Check sheet for the modelled part. Datum: model origin and axes. Units: mm. Face numbers are marked on the shaded views. Give positions to 0.01 mm unless a question says otherwise; leave off trailing zeros. Write each loop counter-clockwise with the first axis right and the second up, starting at its lowest first coordinate (ties: lowest second). Pieces come first, ordered by that corner, then holes. Notation, with made-up numbers: (-35.5, 20.25) -> (15.5, 20.25) arc R28 ccw to (15.5, 49.25) -> close; hole circle Ø1 at (47, 68). An arc over 180 degrees is marked (long way). Return JSON: item names as keys, results as strings.
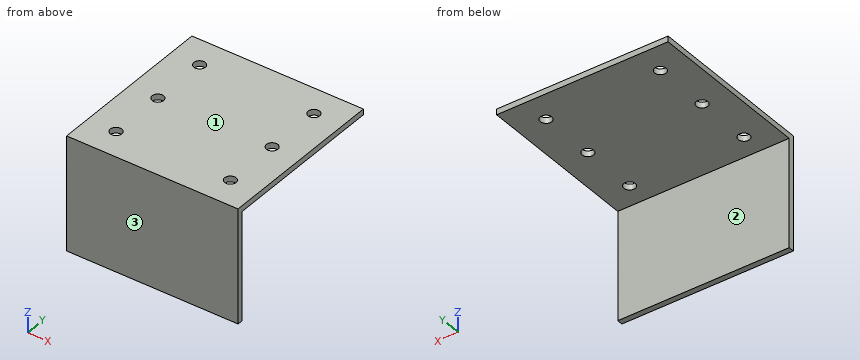
from build123d import *

# Parameters (mm, degrees)
EXTRUDE_1_DEPTH     = 60
SKETCH_2_R          = 2
CUT_EXTRUDE_1_DEPTH = 41


with BuildPart() as part:
    # Эскиз1 → Вытянуть-Тонкостенный1 (new body)
    with BuildSketch(Plane(origin=(0, 0, 0), x_dir=(0, 0, -1), z_dir=(1, 0, 0))):
        Polygon((40, 0), (0, 0), (0, 60), (2, 60), (2, 2), (40, 2), align=None)
    extrude(amount=EXTRUDE_1_DEPTH)

    # Эскиз2 → Вырез-Вытянуть1 (cut, through all)
    with BuildSketch(Plane.XY):
        with Locations((10, 50)):
            Circle(SKETCH_2_R)
        with Locations((50, 50)):
            Circle(SKETCH_2_R)
        with Locations((50, 30)):
            Circle(SKETCH_2_R)
        with Locations((50, 10)):
            Circle(SKETCH_2_R)
        with Locations((10, 30)):
            Circle(SKETCH_2_R)
        with Locations((10, 10)):
            Circle(SKETCH_2_R)
    extrude(amount=-CUT_EXTRUDE_1_DEPTH, mode=Mode.SUBTRACT)


solid = part.part
(1) Thickness scan on L1, parallel to Y at x = 50, z = -1.4; L2, parallel to Y at x = 48.5, z = -32; L3, parallel to Z at x = 48.5, y = 14. Record the ranges inside material, lowest first.
Reply:
{"L1": "0 to 8, 12 to 28, 32 to 48, 52 to 60", "L2": "0 to 2", "L3": "-2 to 0"}
(2) Cross-section at C-C on x = 17.5. Enter the section's corners in (y, z).
Reply:
{"outline": "(0, -40) -> (2, -40) -> (2, -2) -> (60, -2) -> (60, 0) -> (0, 0) -> close"}
(3) Cross-section at A-A on y = 10. Enter the section's corners in (x, z), then the cut area to 3 significant figures.
Reply:
{"outline": "(0, -2) -> (8, -2) -> (8, 0) -> (0, 0) -> close; (12, -2) -> (48, -2) -> (48, 0) -> (12, 0) -> close; (52, -2) -> (60, -2) -> (60, 0) -> (52, 0) -> close", "area": "104 mm^2"}
(4) Cross-section at B-B on x = 50. Enter the section's corners in (y, z), then the cut area to 3 significant figures.
Reply:
{"outline": "(0, -40) -> (2, -40) -> (2, -2) -> (8, -2) -> (8, 0) -> (0, 0) -> close; (12, -2) -> (28, -2) -> (28, 0) -> (12, 0) -> close; (32, -2) -> (48, -2) -> (48, 0) -> (32, 0) -> close; (52, -2) -> (60, -2) -> (60, 0) -> (52, 0) -> close", "area": "172 mm^2"}
(5) Release check for a two-part mould opening along Y. For the marked faces 1, 2 and 3 record: pulls with the +Y half, pulls with the -Y half, needs draft (parallel to the pull), parting line crosses it, or undercut.
Reply:
{"face 1": "needs draft", "face 2": "pulls with the +Y half", "face 3": "pulls with the -Y half"}
(6) Cross-section at D-D on z = -4.5. Enter the section's corners in (x, y), then the cut area to 3 significant figures.
Reply:
{"outline": "(0, 0) -> (60, 0) -> (60, 2) -> (0, 2) -> close", "area": "120 mm^2"}
(7) Depth check by flat-ended pin: pin 1 Ø12 at (x, y) = (16, 10) entering from -Z; pin 2 Ø1.5 at (x, z) = (20, -15.5) entering from +Y. Enter the tip coordinate at first touch or a pass-through.
Reply:
{"pin 1": "z = -2", "pin 2": "y = 2"}
